from build123d import *

# Parameters (mm, degrees)
F0_R          = 19.05
F0_R_2        = 6.35
F1_DEPTH      = 254
F1_DEPTH_BACK = 76.2
F0_R_3        = 63.5
F2_DEPTH      = 12.7


with BuildPart() as f1:
    # F0 (on Right) → F1 (new body, two sides)
    with BuildSketch(Plane.YZ) as f1_sk:
        Circle(F0_R)
        Circle(F0_R_2, mode=Mode.SUBTRACT)
    extrude(amount=-F1_DEPTH)
    extrude(f1_sk.sketch, amount=F1_DEPTH_BACK)

    # F0 (on Right) → F2 (join)
    with BuildSketch(Plane.YZ):
        Circle(F0_R_3)
        Circle(F0_R, mode=Mode.SUBTRACT)
    extrude(amount=-F2_DEPTH)


solid = f1.part
Build history of the part. All positions in model axes, mm. A direction names the side the tool comes from. Coordinates: 2 decimals unless noted, no trailing zeros. Order: outer loops, then holes, each group sorted by start corner. A loop starts at its lowest first (then second) coordinate and runs counter-clockwise, first axis right, second up. Notation, with made-up numbers: M -29.5,21 L 10.5,21 A16 ccw 10.5,37 Z; hole C 73,36 d3. An arc over 180 degrees is marked long. One line per question, with ' | ' between items. Start each with the question number.
Q1. Saw through at C-C (x = -92). List the corners of the cut face in (y, z).
Q2. Flat gauge pins, fed straight in: pin 1 Ø5 at (y, z) = (-41.5, 0.5) entering from +X; pin 2 Ø1 at (x, y) = (4, 6.5) entering from +Z; pin 3 Ø10 at (x, z) = (-86.5, -8.5) entering from +Y. Where does each tip first touch, or does it go through?
Q3. Saw through at D-D (y = 31.5). List the corners of the cut face in (x, z), then the cut area to 3 significant figures.
Q4. Probe L1, parallel to Z at x = -143, y = 0; L2, parallel to X at y = -14.5, z = 52.5; L3, parallel to Y at x = -45, z = 5.5. List the from-to ranges inside material, lowest first. Write a range as from..to.
Q5. Two-plate mould, pull along Z, no slides. Class faces 1 (the face through (-131.66, -15.12, -11.59)), 2 (the face through (76.2, -5, 5)), 3 (the face through (-91.21, -1.38, -6.2)): +Z half, -Z half, draft (parallel to the pull), parting line (faces both ways), or undercut.
Q6. Saw through at A-A (z = 0). List the corners of the cut face in (x, y), then the cut area to 3 significant figures.
Q7. 3-axis set-ups, long thin cutter, end or side, ignore diameter. For faces 4 (the face through (-12.7, 13, 15)), 5 (the face through (-6.26, -13.77, -61.99)), 6 (the face through (0, 13, 15)): which of +Z, -Z, +X, -X, +Y, -Y reach the whole face in a straight line?
Check values:
1) outline: C 0,0 d38.1; hole C 0,0 d12.7
2) pin 1: stops at x = 0 | pin 2: stops at z = 18.08 | pin 3: stops at y = 18.73
3) outline: M -12.7,-55.14 L 0,-55.14 L 0,55.14 L -12.7,55.14 Z | area: 1,400 mm2
4) L1: z = -19.05..-6.35, 6.35..19.05 | L2: x = -12.7..0 | L3: y = -18.24..-3.17, 3.17..18.24
5) face 1: parting line | face 2: draft | face 3: undercut
6) outline: M -254,-19.05 L -12.7,-19.05 L -12.7,-63.5 L 0,-63.5 L 0,-19.05 L 76.2,-19.05 L 76.2,-6.35 L -254,-6.35 Z; M -254,6.35 L 76.2,6.35 L 76.2,19.05 L 0,19.05 L 0,63.5 L -12.7,63.5 L -12.7,19.05 L -254,19.05 Z | area: 9,520 mm2
7) face 4: -X | face 5: +X, -X | face 6: +X
